Geometry: see drawing. Coordinates: mm, zero at the bounding-box minimum. A direction names the side the tool comes from. Give positions to 0.01 mm unless a question says otherwise; leave off trailing zeros. Write each loop counter-clockwise with the first axis right and the second up, starting at its lowest first coordinate (ties: lowest second). Pieces come first, ordered by that corner, then holes. Notation, with made-up numbers: (48.5, 5) -> (57.5, 5) arc R3 ccw to (57.5, 9) -> close; hole circle Ø10 at (-24.5, 49). An arc over 180 degrees is marked (long way). Answer as a JSON object with one key per item and string values. Group by question number.
Item 1: Access query for the marked faces 4, 5 and 6. Directions: +Z, -Z, +X, -X, +Y, -Y. A direction counts if a zero-diameter tool reaches every point of the face in a straight line with its end or side. Return the directions, or none.
Item 2: Pull-direction query (X, two-part tool) for the marked faces 1, 2 and 3; classes: pulls with the +X half, pulls with the -X half, needs draft (parallel to the pull), parting line crosses it, or undercut.
Item 3: First-contact query: pin 1 Ø2.5 at (x, z) = (9.5, 13.5) entering from -Y; pin 2 Ø5 at (y, z) = (4, 18.5) entering from +X; pin 3 Ø6 at (x, z) = (34, 15) entering from +Y; pin 4 Ø4.5 at (x, z) = (35, 12.5) entering from +Y. Flat tips, straight axial feed; report the tip coordinate or a pass-through.
Item 4: Section query B-B on y = 9.75. Return the cut outline in (x, z).
Item 5: Section query C-C on x = 11.5. Return the cut outline in (y, z), plus the area to 3 significant figures.
Item 6: Ray query, probe 1 along Z at (x, y) = (10, 2.9); probe 2 along X at (y, z) = (9.1, 12.5); probe 3 along Z at (x, y) = (35, 11). Return the intervals inside material, ascending. Write a range as from..to.
Item 7: Section query A-A on x = 33. Return the cut outline in (y, z), plus the area to 3 significant figures.
Item 8: Section query D-D on y = 3. Return the cut outline in (x, z), plus the area to 3 significant figures.
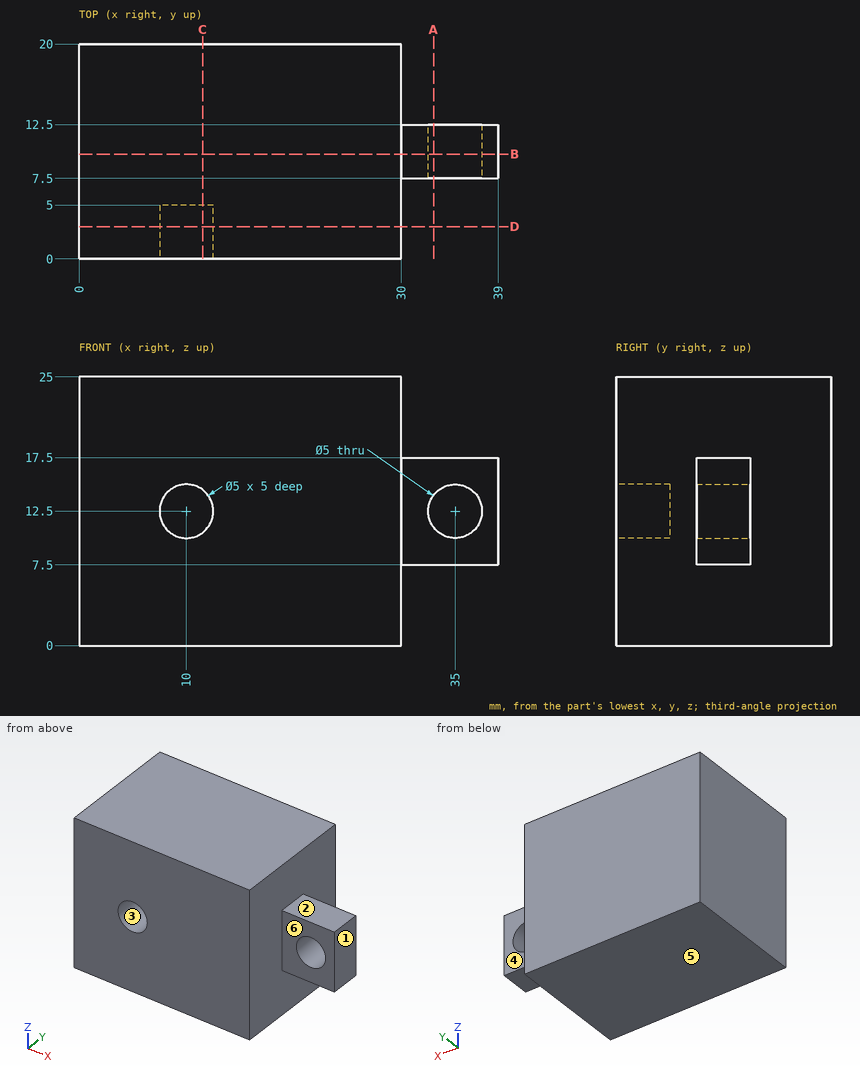
Worked answers:
{
 "1": {"face 4": "+Z, -Z, +X, +Y", "face 5": "-Z, +X, -X, +Y, -Y", "face 6": "+Z, -Z, +X, -Y"},
 "2": {"face 1": "pulls with the +X half", "face 2": "needs draft", "face 3": "undercut"},
 "3": {"pin 1": "y = 5", "pin 2": "x = 30", "pin 3": "y = 12.5", "pin 4": "through"},
 "4": {"outline": "(0, 0) -> (30, 0) -> (30, 7.5) -> (39, 7.5) -> (39, 17.5) -> (30, 17.5) -> (30, 25) -> (0, 25) -> close; hole circle Ø5 at (35, 12.5)"},
 "5": {"outline": "(0, 0) -> (20, 0) -> (20, 25) -> (0, 25) -> (0, 14.5) -> (5, 14.5) -> (5, 10.5) -> (0, 10.5) -> close", "area": "480 mm^2"},
 "6": {"probe 1": "0..10, 15..25", "probe 2": "0..32.5, 37.5..39", "probe 3": "7.5..10, 15..17.5"},
 "7": {"outline": "(7.5, 7.5) -> (12.5, 7.5) -> (12.5, 11) -> (7.5, 11) -> close; (7.5, 14) -> (12.5, 14) -> (12.5, 17.5) -> (7.5, 17.5) -> close", "area": "35.0 mm^2"},
 "8": {"outline": "(0, 0) -> (30, 0) -> (30, 25) -> (0, 25) -> close; hole circle Ø5 at (10, 12.5)", "area": "730 mm^2"}
}
